from build123d import *

# Parameters (mm, degrees)
BOSS_EXTRUDE1_DEPTH     = 45
SKETCH3_R               = 1.7
CUT_EXTRUDE1_DEPTH      = 111.471998715
CHAMFER1_SIZE           = 5
CHAMFER1_SIZE2          = 10
CHAMFER2_SIZE           = 10
CHAMFER2_SIZE2          = 5
FILLET1_R               = 10
CUT_EXTRUDE2_DEPTH      = 112.832743416
CUT_EXTRUDE2_DEPTH_BACK = 112.832743416
SKETCH5_R               = 2.7
CUT_EXTRUDE3_DEPTH      = 112.832743416
CUT_EXTRUDE4_DEPTH      = 20


with BuildPart() as part:
    # Sketch1 → Boss-Extrude1 (new body)
    with BuildSketch(Plane.XY):
        Polygon((0, 0), (0, -5), (-27.75, -5), (-27.75, -25), (-32.75, -25), (-32.75, 97), (-27.75, 97), (-27.75, 57), (0, 57), (0, 52), (-24.5, 52), (-24.5, 0), align=None)
    extrude(amount=BOSS_EXTRUDE1_DEPTH)

    # Sketch3 → Cut-Extrude1 (cut, through all)
    with BuildSketch(Plane(origin=(-27.75, 0, 0), x_dir=(0, 0, -1), z_dir=(1, 0, 0))):
        Polygon((-45, 97), (-45, 82), (-30, 97), align=None)
        Polygon((-15, 97), (0, 82), (0, 97), align=None)
        Polygon((-30, -25), (-45, -15), (-45, -25), align=None)
        Polygon((0, -25), (0, -15), (-15, -25), align=None)
        with Locations(Location((-22.5, -15, 0), (0, 0, 90))):
            Circle(SKETCH3_R)
        with Locations(Location((-22.5, 87, 0), (0, 0, 90))):
            Circle(SKETCH3_R)
        with Locations(Location((-22.5, 67, 0), (0, 0, 90))):
            Circle(SKETCH3_R)
    extrude(amount=-CUT_EXTRUDE1_DEPTH, mode=Mode.SUBTRACT)

    # Chamfer1
    chamfer1_edges = [part.edges().sort_by_distance(p)[0] for p in [
        (-27.75, -5, 22.5),
    ]]
    chamfer1_side = [part.faces().sort_by_distance(p)[0] for p in [
        (-27.75, -10, 0.49244289),
    ]]
    chamfer(chamfer1_edges, length=CHAMFER1_SIZE, length2=CHAMFER1_SIZE2, reference=chamfer1_side[0])

    # Chamfer2
    chamfer2_edges = [part.edges().sort_by_distance(p)[0] for p in [
        (-27.75, 57, 22.5),
    ]]
    chamfer2_side = [part.faces().sort_by_distance(p)[0] for p in [
        (-13.875, 57, 22.5),
    ]]
    chamfer(chamfer2_edges, length=CHAMFER2_SIZE, length2=CHAMFER2_SIZE2, reference=chamfer2_side[0])

    # Fillet1
    fillet1_edges = [part.edges().sort_by_distance(p)[0] for p in [
        (-17.75, 57, 22.5),
        (-30.25, -25, 15),
        (-30.25, -25, 30),
        (-30.25, 97, 15),
        (-30.25, 97, 30),
        (-17.75, -5, 22.5),
    ]]
    fillet(fillet1_edges, radius=FILLET1_R)

    # Sketch5 → Cut-Extrude2 (cut, two sides: drawn at the far end of the back side and taken through both)
    with BuildSketch(Plane(origin=(0, 0, 0), x_dir=(1, 0, 0), z_dir=(0, 1, 0)).offset(-CUT_EXTRUDE2_DEPTH_BACK)):
        with Locations(Location((-11.5, -9.5, 0), (0, 0, 270))):
            Circle(SKETCH5_R)
        with Locations(Location((-11.5, -35.5, 0), (0, 0, 270))):
            Circle(SKETCH5_R)
    extrude(amount=CUT_EXTRUDE2_DEPTH + CUT_EXTRUDE2_DEPTH_BACK, mode=Mode.SUBTRACT)

    # Sketch6 → Cut-Extrude3 (cut, through all)
    with BuildSketch(Plane.XY.offset(45)):
        with BuildLine():
            Line((-24.5, 13), (-29.007418659, 8.563427332))
            ThreePointArc((-29.007418659, 8.563427332), (-30.126939413, 3.104892702), (-25.5, 0))
            Line((-25.5, 0), (-24.5, 0))
            Line((-24.5, 0), (-24.5, 13))
        make_face()
    extrude(amount=-CUT_EXTRUDE3_DEPTH, mode=Mode.SUBTRACT)

    # Sketch7 → Cut-Extrude4 (cut)
    with BuildSketch(Plane.XY.offset(45)):
        with BuildLine():
            Line((-24.5, 18), (-24.5, 34))
            Line((-24.5, 34), (-29.007418659, 29.563427332))
            ThreePointArc((-29.007418659, 29.563427332), (-30.5, 26), (-29.007418659, 22.436572668))
            Line((-29.007418659, 22.436572668), (-24.5, 18))
        make_face()
    extrude(amount=-CUT_EXTRUDE4_DEPTH, mode=Mode.SUBTRACT)


solid = part.part
CAD build for the part. Positions are in the model's coordinates, mm. A direction names the side the tool comes from. Round coordinates to 2 decimals unless told otherwise and drop trailing zeros. Write each loop counter-clockwise with the first axis right and the second up, starting at its lowest first coordinate (ties: lowest second). Pieces come first, ordered by that corner, then holes.
(1) Probe line 1 along Z through (x, y) = (-11.5, 55.95); line 2 along X through (y, z) = (-2.8, 35.5); line 3 along Y through (x, z) = (-10, 12.5). List the from-to ranges inside material, lowest first.
(2) Mould opens along Y. For faces 1 (the face through (-26, 30, 0)), 2 (the face through (-27, 26, 25)), 3 (the face through (-30.28, -24.56, 15.09)), 4 (the face through (-30.22, 65.3, 22.57)) say: pulls with the +Y half, pulls with the -Y half, needs draft (parallel to the pull), parting line crosses it, or undercut.
(3) Drop flat-ended pins along their axis: P1, Ø8.5, axis at x = -11.5, z = 9.5, coming from the +Y side; P2, Ø2.5, axis at y = 67, z = 22.5, coming from the -X side; P3, Ø7.5, axis at x = -5.5, z = 32, coming from the -Y side; P4, Ø1, axis at x = -27.5, z = 6.5, coming from the +Y side. Give the stop position or say it passes through.
(4) Slice it at D-D, the plane z = 35.5. Count the separate pieces of the cut face and the enclosed holes in it, and give its area (3 significant figures).
(5) Slice it at C-C, the plane x = -11.5. Write the cut outline in (y, z), and give its area (3 significant figures).
(6) 3-axis set-ups, long thin cutter, end or side, ignore diameter. For faces 5 (the face through (-8, -5, 22)), 6 (the face through (-27.75, 76, 22)), 7 (the face through (-26.722, 31.813, 35.14)): which of +Z, -Z, +X, -X, +Y, -Y reach the whole face in a straight line?
(7) Slice it at B-B, the plane y = 67. Write the cut outline in (x, z), and give its area (3 significant figures).
(8) Slice it at A-A, the plane x = -5.5. Write the cut outline in (y, z), and give its area (3 significant figures).
From the geometry:
1. line 1: z = 0 to 6.8, 12.2 to 32.8, 38.2 to 45
1. line 2: x = -32.75 to -14.2, -8.8 to 0
1. line 3: y = -5 to 0, 52 to 57
2. face 1: needs draft
2. face 2: undercut
2. face 3: pulls with the -Y half
2. face 4: undercut
3. P1: stops at y = 57.01
3. P2: passes through
3. P3: stops at y = -5
3. P4: stops at y = 88.93
4. separate pieces: 3
4. enclosed holes: 0
4. area: 894 mm2
5. outline: (-5, 0) - (0, 0) - (0, 6.8) - (-5, 6.8) - close; (-5, 12.2) - (0, 12.2) - (0, 32.8) - (-5, 32.8) - close; (-5, 38.2) - (0, 38.2) - (0, 45) - (-5, 45) - close; (52, 0) - (57, 0) - (57, 6.8) - (52, 6.8) - close; (52, 12.2) - (57, 12.2) - (57, 32.8) - (52, 32.8) - close; (52, 38.2) - (57, 38.2) - (57, 45) - (52, 45) - close
5. area: 342 mm2
6. face 5: +Z, -Z, +X, -Y
6. face 6: +Z, -Z, +X, +Y
6. face 7: +Z, +X
7. outline: (-32.75, 0) - (-27.75, 0) - (-27.75, 20.8) - (-32.75, 20.8) - close; (-32.75, 24.2) - (-27.75, 24.2) - (-27.75, 45) - (-32.75, 45) - close
7. area: 208 mm2
8. outline: (-5, 0) - (0, 0) - (0, 45) - (-5, 45) - close; (52, 0) - (57, 0) - (57, 45) - (52, 45) - close
8. area: 450 mm2
